Job drawing, mm, ordinate dimensions from the low corner. One solid piece. A direction names the side the tool comes from. Give positions to 0.01 mm unless a question says otherwise; leave off trailing zeros. Loops run counter-clockwise (first coordinate to the right, second up) from the corner with the lowest first, then second, coordinate; pieces in that order, holes last. Notation, with made-up numbers: (61.25, 49) -> (73.25, 49) arc R10 cw to (73.25, 57) -> close; hole circle Ø8 at (81, 16.25). An arc over 180 degrees is marked (long way). Use one line per item in the form item = value.
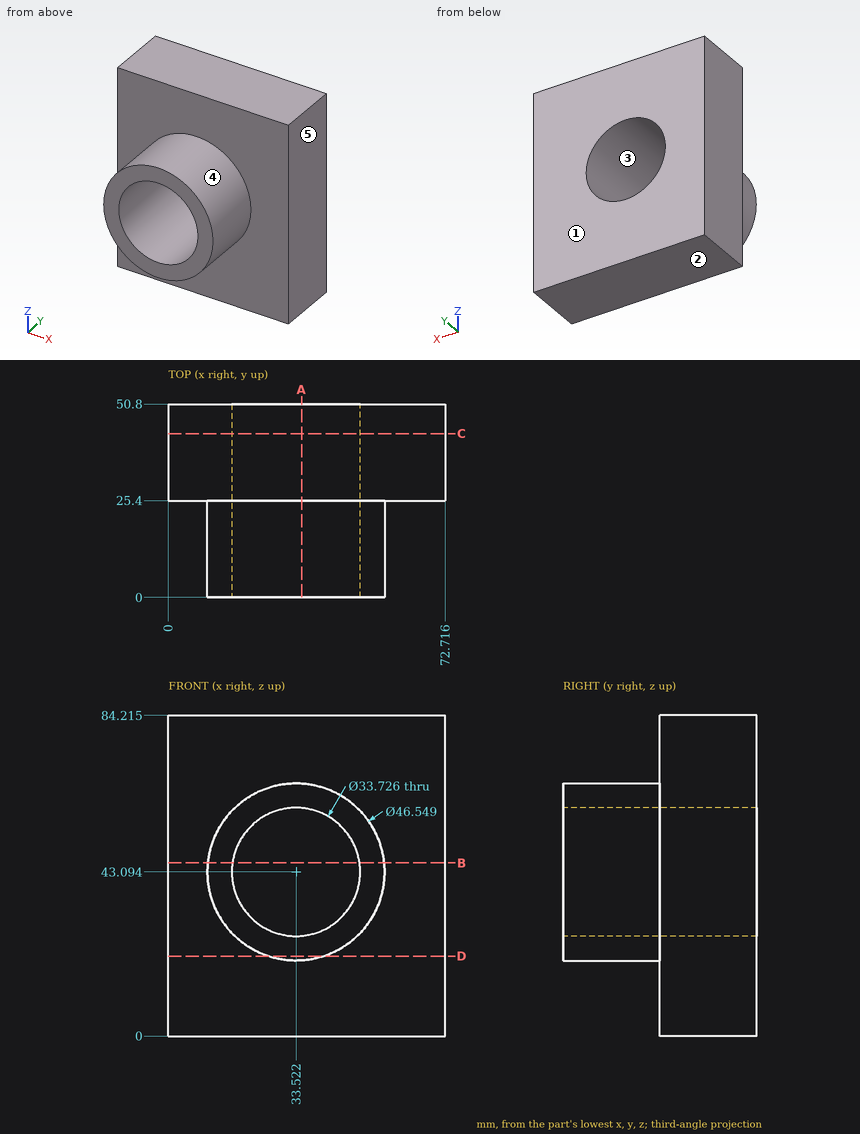
1. Drill centre lines: line 1 (Y direction, x = 37, z = 8); line 2 (Z direction, x = 30, y = 30) (1 decimal); line 3 (X direction, y = 17, z = 58.5) (1 decimal). Where is each one in solid material? Low to high.
Result sheet:
line_1 = 25.4 to 50.8
line_2 = 0 to 26.6, 59.6 to 84.2
line_3 = 16.1 to 26.7, 40.4 to 51
2. Mould opens along Z. For the marked faces 1, 2 and 3 say: pulls with the +Z half, pulls with the -Z half, needs draft (parallel to the pull), parting line crosses it, or undercut.
Result sheet:
face_1 = needs draft
face_2 = pulls with the -Z half
face_3 = undercut
3. Tool access for the marked faces 4 and 5: list every direction of +Z, -Z, +X, -X, +Y, -Y with a clear straight run to the whole face (end or side of a thin tool).
Result sheet:
face_4 = -Y
face_5 = +Z, -Z, +X, +Y, -Y
4. Cut at C-C, the plane y = 43. Write the cut outline in (x, z) (1 decimal), then the cut area to 3 significant figures.
Result sheet:
outline = (0, 0) -> (72.7, 0) -> (72.7, 84.2) -> (0, 84.2) -> close; hole circle Ø33.7 at (33.5, 43.1)
area = 5,230 mm^2
5. Cut at A-A, the plane x = 35. Write the cut outline in (y, z) (1 decimal), then the cut area to 3 significant figures.
Result sheet:
outline = (0, 19.9) -> (25.4, 19.9) -> (25.4, 0) -> (50.8, 0) -> (50.8, 26.3) -> (0, 26.3) -> close; (0, 59.9) -> (50.8, 59.9) -> (50.8, 84.2) -> (25.4, 84.2) -> (25.4, 66.3) -> (0, 66.3) -> close
area = 1,610 mm^2
6. Drop flat-ended pins along their axis: P1, Ø5, axis at x = 24, y = 16, coming from the +Z side; P2, Ø8, axis at y = 8.5, z = 62.5, coming from the +X side. Give the stop position or say it passes through.
Result sheet:
P1 = 65.28
P2 = 50.97
7. Cut at D-D, the plane z = 21. Write the cut outline in (x, y), then the cut area to 3 significant figures.
Result sheet:
outline = (0, 25.4) -> (26.2, 25.4) -> (26.2, 0) -> (40.84, 0) -> (40.84, 25.4) -> (72.72, 25.4) -> (72.72, 50.8) -> (0, 50.8) -> close
area = 2,220 mm^2
8. Cut at B-B, the plane z = 45.5. Write the cut outline in (x, y), then the cut area to 3 significant figures.
Result sheet:
outline = (0, 25.4) -> (10.37, 25.4) -> (10.37, 0) -> (16.83, 0) -> (16.83, 50.8) -> (0, 50.8) -> close; (50.21, 0) -> (56.67, 0) -> (56.67, 25.4) -> (72.72, 25.4) -> (72.72, 50.8) -> (50.21, 50.8) -> close
area = 1,330 mm^2
